Print and shaded views of the part. All mm, measured from the part's lowest x, y and z. Coordinates: 2 decimals unless noted, no trailing zeros. Write each loop counter-clockwise with the first axis right and the second up, starting at its lowest first coordinate (ties: lowest second). Pieces come first, ordered by that corner, then holes. Notation, with made-up numbers: (-25, 31) -> (3, 31) arc R13 cw to (3, 40) -> close; hole circle Ø9 at (-16.75, -8). An arc over 180 degrees is marked (long way). Write item = value, one per line.
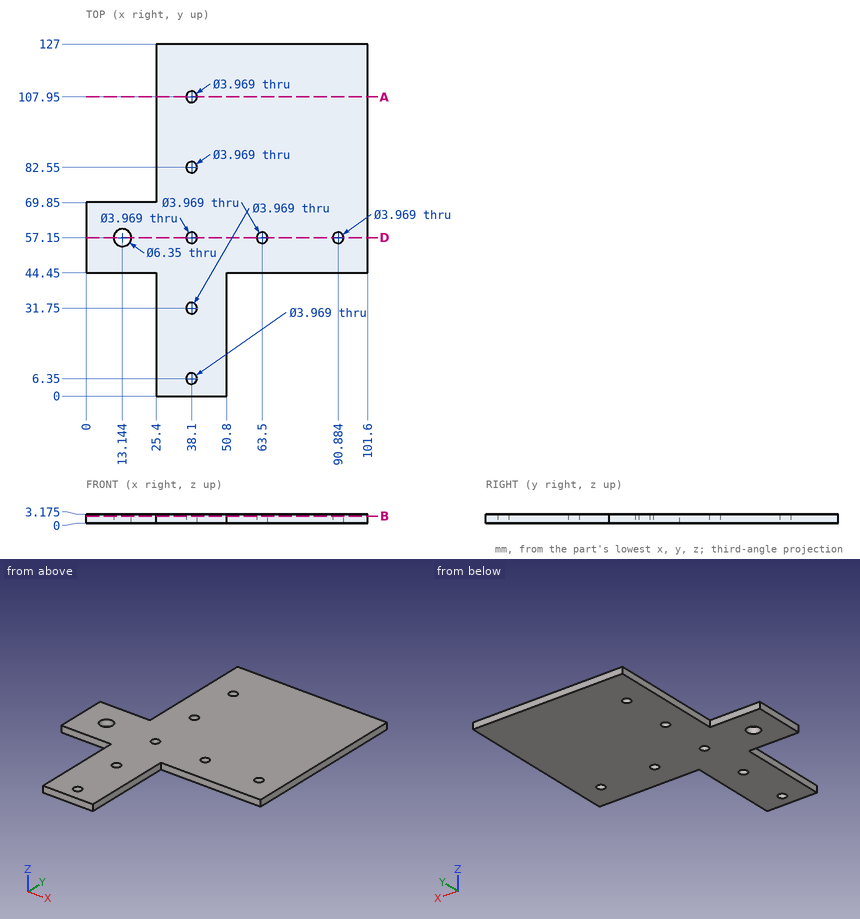
Q1. Pin check, flat tips, straight feed: pin 1 (1 mm diameter, centred on x = 16, z = 2.5, fed in from -Y); pin 2 (1.6 mm diameter, centred on y = 85, z = 1.5, fed in from -X); pin 3 (5 mm diameter, centred on x = 38.1, y = 57.15, fed in from +Z) (3 decimals); pin 4 (1 mm diameter, centred on x = 15.5, z = 1.5, fed in from +Y). Stop position of each tip, or through.
Model answer:
pin_1 = 44.45
pin_2 = 25.4
pin_3 = 3.175
pin_4 = 69.85
Q2. Saw through at B-B on z = 2.45. Count the separate pieces of the cut face and the enclosed holes in it, and give its area (3 significant figures).
Model answer:
separate_pieces = 1
enclosed_holes = 8
area = 7,950 mm²
Q3. Saw through at A-A on y = 107.95. Give the cut face in (x, z) (1 decimal).
Model answer:
outline = (25.4, 0) -> (36.1, 0) -> (36.1, 3.2) -> (25.4, 3.2) -> close; (40.1, 0) -> (101.6, 0) -> (101.6, 3.2) -> (40.1, 3.2) -> close
Q4. Probe line 1 (Y direction, x = 38.1, z = 1.35) (1 decimal); line 2 (X direction, y = 6, z = 2.5); line 3 (Y direction, x = 20.5, z = 0.2). List the from-to ranges inside material, lowest first. Write a range as from..to.
Model answer:
line_1 = 0..4.4, 8.3..29.8, 33.7..55.2, 59.1..80.6, 84.5..106, 109.9..127
line_2 = 25.4..36.15, 40.05..50.8
line_3 = 44.45..69.85
Q5. Saw through at D-D on y = 57.15. Give the cut face in (x, z) (1 decimal).
Model answer:
outline = (0, 0) -> (10, 0) -> (10, 3.2) -> (0, 3.2) -> close; (16.3, 0) -> (36.1, 0) -> (36.1, 3.2) -> (16.3, 3.2) -> close; (40.1, 0) -> (61.5, 0) -> (61.5, 3.2) -> (40.1, 3.2) -> close; (65.5, 0) -> (88.9, 0) -> (88.9, 3.2) -> (65.5, 3.2) -> close; (92.9, 0) -> (101.6, 0) -> (101.6, 3.2) -> (92.9, 3.2) -> close
